Could you check a few things on this model? Use its own coordinates, in mm. Face numbers are marked on the shaded views. A direction names the side the tool comes from. Round coordinates to 2 decimals unless told otherwise and drop trailing zeros. Write each loop counter-clockwise with the first axis right and the second up, starting at its lowest first coordinate (ties: lowest second). Pieces come first, ordered by that corner, then holes. Notation, with made-up numbers: (88.5, -24.5) -> (102.5, -24.5) arc R18 ccw to (102.5, 6.5) -> close; hole circle Ø7 at (77, 79.5). An arc over 180 degrees is marked (long way). Answer in a Markdown table with one row per item.
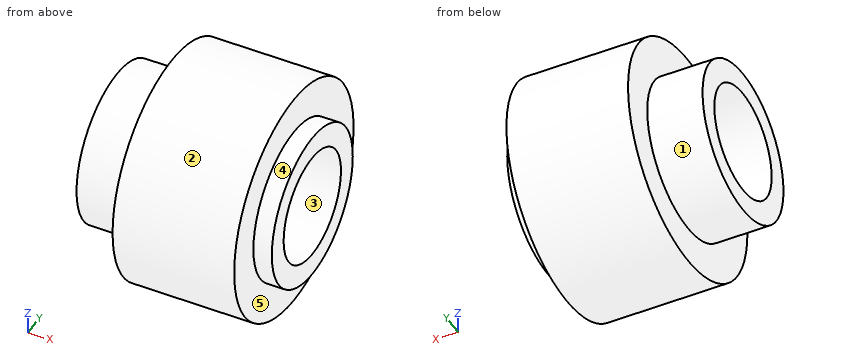
Autodesk Inventor part; units mm, degrees
ref_plane "YZ Plane" through (0, 0, 0) normal (1, 0, 0) x (0, 1, 0)
ref_plane "XZ Plane" through (0, 0, 0) normal (0, 1, 0) x (-1, 0, 0)
ref_plane "XY Plane" through (0, 0, 0) normal (0, 0, 1) x (1, 0, 0)
sketch "Boceto6" plane through (0, 0, 0) normal (1, 0, 0) x (0, 1, 0)
  circle A0 centre (0, 0) radius 6
  circle A1 centre (0, 0) radius 12.5
  circle A2 centre (0, 0) radius 8.475
  dimension "d16" = 12
  dimension "d17" = 25
  dimension "d18" = 16.95
extrude "Extrusión6" add sketch "Boceto6" along normal blind 4 and the other way blind 4 contours A1
extrude "Extrusión7" add sketch "Boceto6" along normal blind 6.2 and the other way blind 10 contours A2
sketch "Boceto7" plane through (4, 0, 0) normal (1, 0, 0) x (0, 0, -1)
  circle A0 centre (0, 0) radius 6
  circle A1 centre (0, 0) radius 8.475
  circle A2 centre (0, 0) radius 12.5
extrude "Extrusión8" add sketch "Boceto7" along normal blind 5.2 contours A2
extrude "Extrusión9" add sketch "Boceto7" along normal blind 7.2 contours A1
properties part number "Buge"
1) Imagine slicing it at A-A, the plane y = 0. Please give me the cut outline in (x, z) (3 decimals), plus the area to 3 significant figures.
Findings:
| item | result |
|---|---|
| outline | (-10, -8.475) -> (-4, -8.475) -> (-4, -12.5) -> (9.2, -12.5) -> (9.2, -8.475) -> (11.2, -8.475) -> (11.2, -6) -> (-10, -6) -> close; (-10, 6) -> (11.2, 6) -> (11.2, 8.475) -> (9.2, 8.475) -> (9.2, 12.5) -> (-4, 12.5) -> (-4, 8.475) -> (-10, 8.475) -> close |
| area | 211 mm^2 |
2) Imagine slicing it at C-C, the plane x = -3. Please give me the cut outline in (y, z).
Findings:
| item | result |
|---|---|
| outline | circle Ø25 at (0, 0); hole circle Ø12 at (0, 0) |
3) Please list where these lines run through material, in increasing order: line 1 (Y direction, x = -3.25, z = 0); line 2 (X direction, y = 3, z = -11.5).
Findings:
| item | result |
|---|---|
| line 1 | y = -12.5 to -6, 6 to 12.5 |
| line 2 | x = -4 to 9.2 |
4) Thinking about a two-plate mould opening in Z: for the marked faces 3, 4 and 5, which applies, +Z half, -Z half, draft (parallel to the pull), parting line (faces both ways), or undercut?
Findings:
| item | result |
|---|---|
| face 3 | undercut |
| face 4 | parting line |
| face 5 | draft |
5) Imagine slicing it at D-D, the plane y = 10.5. Please give me the cut outline in (x, z), plus the area to 3 significant figures.
Findings:
| item | result |
|---|---|
| outline | (-4, -6.78) -> (9.2, -6.78) -> (9.2, 6.78) -> (-4, 6.78) -> close |
| area | 179 mm^2 |
6) For the marked faces 1 and 2, which set-ups out of +Z, -Z, +X, -X, +Y, -Y let a thin tool reach every point of the face, with its end or its side?
Findings:
| item | result |
|---|---|
| face 1 | -X |
| face 2 | +X, -X |
7) For pin 1 (2 mm diameter, centred on y = -7, z = -8, fed in from -X); pin 2 (4 mm diameter, centred on x = 6.5, y = -8, fed in from -Z); pin 3 (6 mm diameter, centred on x = -1, z = -7, fed in from +Y), each with a flat end and sliding along its axis, tell me the tip position at first contact or that it passes through.
Findings:
| item | result |
|---|---|
| pin 1 | stops at x = -4 |
| pin 2 | stops at z = -10.97 |
| pin 3 | stops at y = 11.84 |
